Autodesk Inventor part; units mm, degrees
ref_plane "YZ Plane" through (0, 0, 0) normal (1, 0, 0) x (0, 1, 0)
ref_plane "XZ Plane" through (0, 0, 0) normal (0, 1, 0) x (-1, 0, 0)
ref_plane "XY Plane" through (0, 0, 0) normal (0, 0, 1) x (1, 0, 0)
sketch "Sketch2" plane through (0, 0, 0) normal (0, 1, 0) x (-1, 0, 0)
  line L0 (215.9, 254) -> (-215.9, 254)
  line L1 (-215.9, 254) -> (-215.9, -254)
  line L2 (-215.9, -254) -> (215.9, -254)
  line L3 (215.9, -254) -> (215.9, 254)
  line L4 (215.9, 254) -> (-215.9, -254) construction
  line L5 (-215.9, 254) -> (215.9, -254) construction
  point P0 (0, 0)
  point P1 (0, -254)
  dimension "d6" = 431.8
  dimension "d7" = 508
extrude "Extrusion3" add sketch "Sketch2" along normal blind 133.35
ref_plane "Work Plane3" through (0, 133.35, 254) normal (1, 0, 0) x (0, 1, 0)
sketch "Sketch4" plane through (0, 133.35, 0) normal (0, 1, 0) x (1, 0, 0)
  line L0 (-215.9, -254) -> (215.9, -254)
  line L1 (215.9, -228.6) -> (215.9, -254)
  line L2 (215.9, -254) -> (241.3, -254)
  line L3 (241.3, -251.3584) -> (218.5416, -251.3584)
  line L4 (218.5416, -251.3584) -> (218.5416, -228.6)
  line L5 (215.9, -228.6) -> (218.5416, -228.6)
  line L6 (215.9, -254) -> (215.9, 254)
  line L7 (241.3, -254) -> (241.3, -251.3584)
  point P0 (0, 0)
  dimension "d13" = 25.4
  dimension "d14" = 25.4
  dimension "d15" = 2.6416
extrude "Extrusion5" add sketch "Sketch4" against normal blind 133.35
mirror "Mirror1" about plane through (0, 133.35, 254) normal (1, 0, 0) of "Extrusion5"
equation "\"BendRadius\" = Thickness"
equation "\"BendReliefWidth\" = Thickness"
equation "\"BendReliefDepth\" = 0.5 * Thickness"
equation "\"CornerReliefSize\" = 4 * Thickness"
equation "\"MinimumRemnant\" = 2 * Thickness"
equation "\"TransitionRadius\" = BendRadius"
equation "\"JacobiRadiusSize\" = Thickness"
equation "\"GapSize\" = Thickness"
properties part number "powerDistribution"
Verification items for the finished model (mm, model axes). A direction names the side the tool comes from. Give positions to 0.01 mm unless a question says otherwise; leave off trailing zeros. Order: outer loops, then holes, each group sorted by start corner. A loop starts at its lowest first (then second) coordinate and runs counter-clockwise, first axis right, second up. Notation, with made-up numbers: M 11.25,64 L 56.25,64 A26 ccw 56.25,89 Z; hole C 49.25,47 d8. An arc over 180 degrees is marked long. Return JSON: item names as keys, results as strings. Group by question number.
1) Section check B-B on z = -74. Record the cut outline in (x, y).
2) Go/stop test with flat-tipped pins: pin 1 Ø18 at (x, y) = (-234.5, 44.5) entering from -Z; pin 2 Ø1.5 at (y, z) = (45.5, -126) entering from +X; pin 3 Ø0.8 at (x, y) = (217.5, 67) entering from -Z. Record where each tip stops, or that it passes through.
3) Section check A-A on y = 121.5. Record the cut outline in (x, z).
4) Scan lines: line 1 (X direction, y = 19, z = -33); line 2 (Z direction, x = 216, y = 15). Record each from-to range of solid material in increasing order.
5) Access from +Z, -Z, +X, -X, +Y, -Y to the whole of each face (thin tool, end or side, straight path). Record for faces 1 (the face through (-230, 68, 251.358)), 2 (the face through (3, 66, -254)), 3 (the face through (218.542, 68, 240)).
Answer block:
{
 "1": {"outline": "M -215.9,0 L 215.9,0 L 215.9,133.35 L -215.9,133.35 Z"},
 "2": {"pin 1": "stops at z = 251.36", "pin 2": "stops at x = 215.9", "pin 3": "stops at z = 228.6"},
 "3": {"outline": "M -241.3,251.36 L -218.54,251.36 L -218.54,228.6 L -215.9,228.6 L -215.9,-254 L 215.9,-254 L 215.9,228.6 L 218.54,228.6 L 218.54,251.36 L 241.3,251.36 L 241.3,254 L -241.3,254 Z"},
 "4": {"line 1": "x = -215.9 to 215.9", "line 2": "z = 228.6 to 254"},
 "5": {"face 1": "-Z, -X, +Y, -Y", "face 2": "-Z, +X, -X, +Y, -Y", "face 3": "-Z, +X, +Y, -Y"}
}
